Read the model definition and answer for the solid it produces. Units are mm, in the model's axes. Coordinates: 2 decimals unless noted, no trailing zeros. Write each loop counter-clockwise with the first axis right and the second up, starting at its lowest first coordinate (ties: lowest second). Pieces come first, ordered by that corner, then holes. Notation, with made-up numbers: (-10, -9) -> (-5, -9) arc R22 cw to (-5, 26) -> close; hole circle Ø9 at (-10.5, 31.25). An arc over 180 degrees is marked (long way). Answer in a Markdown table with one row per item. Add a question column.
Item 1: Section D-D on x = 13 is taken. Write down the section's boundary in (y, z) (1 decimal).
Item 2: Straight lines are drawn through the part: line 1 (Z direction, x = 7.5, y = 21.25); line 2 (X direction, y = 21, z = 6.5); line 3 (X direction, y = 20, z = 14.5). For each, find the intervals that lie inside material, in ascending order. Write a range as from..to.
Item 3: Section B-B on y = 8 is taken. Write down the section's boundary in (x, z) (3 decimals).
Item 4: Section C-C on z = 22 is taken. Write down the section's boundary in (x, y).
Item 5: Given pin 1 Ø1.5 at (y, z) = (17, -3.5) entering from -X; pin 2 Ø4 at (y, z) = (7.5, 19) entering from +X, each flat-ended and moving along its own axis, determine where each tip first touches the part or whether it passes through.
Item 6: Section A-A on x = 3.5 is taken. Write down the section's boundary in (y, z) (1 decimal).
```python
from build123d import *

# Parameters (mm, degrees)
BOSS_EXTRUDE1_DEPTH = 25.4
FILLET1_R           = 4.7625


with BuildPart() as part:
    # Sketch1 → Boss-Extrude1 (new body)
    with BuildSketch(Plane(origin=(0, 0, 0), x_dir=(1, 0, 0), z_dir=(0, 1, 0))):
        with BuildLine():
            Line((0, -25.4), (0, 25.4))
            Line((0, 25.4), (9.525, 25.4))
            ThreePointArc((9.525, 25.4), (11.118653193, -0.197668351), (15.875, -25.4))
            Line((15.875, -25.4), (0, -25.4))
        make_face()
    extrude(amount=BOSS_EXTRUDE1_DEPTH)

    # Fillet1
    fillet1_edges = [part.edges().sort_by_distance(p)[0] for p in [
        (7.9375, 25.4, 25.4),
        (4.7625, 25.4, -25.4),
        (7.9375, 0, 25.4),
        (4.7625, 0, -25.4),
    ]]
    fillet(fillet1_edges, radius=FILLET1_R)


solid = part.part
```
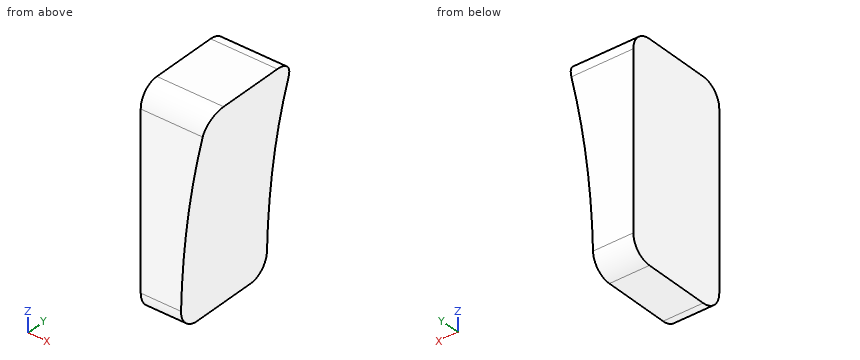
Results below:
| question | item | result |
|---|---|---|
| 1 | outline | (0, 12.3) -> (25.4, 12.3) -> (25.4, 20.6) arc R4.8 ccw to (20.6, 25.4) -> (4.8, 25.4) arc R4.8 ccw to (0, 20.6) -> close |
| 2 | line 1 | z = -25.36..25.36 |
| 2 | line 2 | x = 0..12.01 |
| 2 | line 3 | x = 0..13.42 |
| 3 | outline | (0, -25.4) -> (9.525, -25.4) arc R206.375 cw to (15.875, 25.4) -> (0, 25.4) -> close |
| 4 | outline | (0, 0.2) -> (15.04, 0.2) -> (15.04, 25.2) -> (0, 25.2) -> close |
| 5 | pin 1 | stops at x = 0 |
| 5 | pin 2 | stops at x = 14.81 |
| 6 | outline | (0, -20.6) arc R4.8 ccw to (4.8, -25.4) -> (20.6, -25.4) arc R4.8 ccw to (25.4, -20.6) -> (25.4, 20.6) arc R4.8 ccw to (20.6, 25.4) -> (4.8, 25.4) arc R4.8 ccw to (0, 20.6) -> close |
